Read the model definition and answer for the solid it produces. Units are mm, in the model's axes. A direction names the side the tool comes from. Round coordinates to 2 decimals unless told otherwise and drop trailing zeros. Order: outer loops, then holes, each group sorted by start corner. A loop starts at its lowest first (then second) coordinate and runs counter-clockwise, first axis right, second up. Notation, with made-up numbers: (50, -20) -> (81, -20) arc R29 cw to (81, 18) -> close; hole circle Ø10 at (5.5, -16). An arc over 180 degrees is marked (long way). Use a Markdown table: item, result. Add a question column.
1. Section C-C, the plane z = 9.5 is taken. Give the vertices of the cut face in (x, y), then the cut area to 3 significant figures.
2. Given pin 1 (1 mm diameter, centred on x = 64, y = 2.5, fed in from +Z); pin 2 (2 mm diameter, centred on x = 5, y = 3, fed in from +Z); pin 3 (1 mm diameter, centred on x = 7, y = 2, fed in from -Z), each flat-ended and moving along its own axis, determine where each tip first touches the part or whether it passes through.
3. The mould has two halves that part along Z. Classify faces 5 (the face through (12, 3.7, 27)), 6 (the face through (39, 1.2, 18)), 7 (the face through (41, 2, 31)), 8 (the face through (64.1, 0.61, 0.86)): +Z half, -Z half, draft (parallel to the pull), parting line (faces both ways), or undercut.
4. Section A-A, the plane z = 21 is taken. Give the vertices of the cut face in (x, y), then the cut area to 3 significant figures.
5. Consider L1, parallel to Z at x = 3.5, y = 0.75; L2, parallel to X at y = 0.95, z = 3.5; L3, parallel to Z at x = 13, y = 1.7. Determine where each line is inside the solid, lowest interval first. Write a range as [from, to].
6. Section B-B, the plane x = 56 is taken. Give the vertices of the cut face in (y, z), then the cut area to 3 significant figures.
7. Section D-D, the plane z = 6 is taken. Give the vertices of the cut face in (x, y).
8. For faces 1 (the face through (0.86, 0.61, 0.9)), 2 (the face through (63, 2, 7)), 3 (the face through (61, 2, 15)), 4 (the face through (37.4, 2, 28)), determine the directions among +Z, -Z, +X, -X, +Y, -Y from which every point of the face is accessible in a straight line to the end or side of a thin tool.
```python
from build123d import *

# Parameters (mm, degrees)
SKETCH1_W           = 65
SKETCH1_H           = 30
BOSS_EXTRUDE1_DEPTH = 1.2
SKETCH2_R           = 1.5
CUT_EXTRUDE1_DEPTH  = 2.2
FILLET1_R           = 3
SKETCH3_W           = 12
SKETCH3_H           = 12.2
BOSS_EXTRUDE2_DEPTH = 1.2
SKETCH4_W           = 11.8
SKETCH4_H           = 1.2
BOSS_EXTRUDE3_DEPTH = 5
SKETCH5_W           = 12
SKETCH5_H           = 7
BOSS_EXTRUDE4_DEPTH = 2.5
SKETCH6_W           = 8
SKETCH6_H           = 6
BOSS_EXTRUDE5_DEPTH = 2.5
SKETCH7_W           = 5
SKETCH7_H           = 16
BOSS_EXTRUDE6_DEPTH = 2
SKETCH8_W           = 52
SKETCH8_H           = 4
BOSS_EXTRUDE7_DEPTH = 1


with BuildPart() as part:
    # Sketch1 → Boss-Extrude1 (new body)
    with BuildSketch(Plane(origin=(0, 0, 0), x_dir=(1, 0, 0), z_dir=(0, 1, 0))):
        with Locations((32.5, -15)):
            Rectangle(SKETCH1_W, SKETCH1_H)
    extrude(amount=BOSS_EXTRUDE1_DEPTH)

    # Sketch2 → Cut-Extrude1 (cut, through all)
    with BuildSketch(Plane(origin=(0, 1.2, 0), x_dir=(1, 0, 0), z_dir=(0, 1, 0))):
        with Locations((3.5, -26.5)):
            Circle(SKETCH2_R)
        with Locations((61.5, -26.5)):
            Circle(SKETCH2_R)
        with Locations((61.5, -3.5)):
            Circle(SKETCH2_R)
        with Locations((3.5, -3.5)):
            Circle(SKETCH2_R)
    extrude(amount=-CUT_EXTRUDE1_DEPTH, mode=Mode.SUBTRACT)

    # Fillet1
    fillet1_edges = [part.edges().sort_by_distance(p)[0] for p in [
        (0, 0.6, 0),
        (65, 0.6, 0),
        (65, 0.6, 30),
        (0, 0.6, 30),
    ]]
    fillet(fillet1_edges, radius=FILLET1_R)

    # Sketch3 → Boss-Extrude2 (add)
    with BuildSketch(Plane(origin=(0, 1.2, 0), x_dir=(1, 0, 0), z_dir=(0, 1, 0))):
        with Locations((7.5, -13.1)):
            Rectangle(SKETCH3_W, SKETCH3_H)
    extrude(amount=BOSS_EXTRUDE2_DEPTH)

    # Sketch4 → Boss-Extrude3 (add)
    with BuildSketch(Plane.ZY.offset(-1.5)):
        with Locations((13.1, 1.8)):
            Rectangle(SKETCH4_W, SKETCH4_H)
    extrude(amount=BOSS_EXTRUDE3_DEPTH)

    # Sketch5 → Boss-Extrude4 (add)
    with BuildSketch(Plane(origin=(0, 1.2, 0), x_dir=(1, 0, 0), z_dir=(0, 1, 0))):
        with Locations((12.4, -26.8)):
            Rectangle(SKETCH5_W, SKETCH5_H)
    extrude(amount=BOSS_EXTRUDE4_DEPTH)

    # Sketch6 → Boss-Extrude5 (add)
    with BuildSketch(Plane(origin=(0, 1.2, 0), x_dir=(1, 0, 0), z_dir=(0, 1, 0))):
        with Locations((41.4, -28)):
            Rectangle(SKETCH6_W, SKETCH6_H)
        with Locations((54, -28)):
            Rectangle(SKETCH6_W, SKETCH6_H)
    extrude(amount=BOSS_EXTRUDE5_DEPTH)

    # Sketch7 → Boss-Extrude6 (add)
    with BuildSketch(Plane(origin=(0, 1.2, 0), x_dir=(1, 0, 0), z_dir=(0, 1, 0))):
        with Locations((63.5, -15)):
            Rectangle(SKETCH7_W, SKETCH7_H)
    extrude(amount=BOSS_EXTRUDE6_DEPTH)

    # Sketch8 → Boss-Extrude7 (add)
    with BuildSketch(Plane(origin=(0, 1.2, 0), x_dir=(1, 0, 0), z_dir=(0, 1, 0))):
        with Locations((32.5, -3)):
            Rectangle(SKETCH8_W, SKETCH8_H)
    extrude(amount=BOSS_EXTRUDE7_DEPTH)


solid = part.part
```
Verdict:
| question | item | result |
|---|---|---|
| 1 | outline | (-3.5, 1.2) -> (0, 1.2) -> (0, 0) -> (65, 0) -> (65, 1.2) -> (66, 1.2) -> (66, 3.2) -> (61, 3.2) -> (61, 1.2) -> (13.5, 1.2) -> (13.5, 2.4) -> (-3.5, 2.4) -> close |
| 1 | area | 108 mm2 |
| 2 | pin 1 | stops at z = 23 |
| 2 | pin 2 | stops at z = 19.2 |
| 2 | pin 3 | stops at z = 1 |
| 3 | face 5 | draft |
| 3 | face 6 | undercut |
| 3 | face 7 | +Z half |
| 3 | face 8 | -Z half |
| 4 | outline | (0, 0) -> (65, 0) -> (65, 1.2) -> (66, 1.2) -> (66, 3.2) -> (61, 3.2) -> (61, 1.2) -> (0, 1.2) -> close |
| 4 | area | 88.0 mm2 |
| 5 | L1 | z = [0, 2], [5, 25], [28, 30] |
| 5 | L2 | x = [0, 2], [5, 60], [63, 65] |
| 5 | L3 | z = [1, 5], [7, 19.2], [23.3, 30.3] |
| 6 | outline | (0, 0) -> (1.2, 0) -> (1.2, 1) -> (2.2, 1) -> (2.2, 5) -> (1.2, 5) -> (1.2, 25) -> (3.7, 25) -> (3.7, 31) -> (1.2, 31) -> (1.2, 30) -> (0, 30) -> close |
| 6 | area | 55.0 mm2 |
| 7 | outline | (0, 0) -> (65, 0) -> (65, 1.2) -> (0, 1.2) -> close |
| 8 | face 1 | -Z, -X, +Y, -Y |
| 8 | face 2 | -Z, +X, -X, +Y |
| 8 | face 3 | +Z, -Z, +Y |
| 8 | face 4 | +Z, +Y |
